The model under review builds one solid part; all positions refer to its coordinate system, in mm. A direction names the side the tool comes from. Round coordinates to 2 decimals unless told otherwise and drop trailing zeros. Loops run counter-clockwise (first coordinate to the right, second up) from the corner with the lowest first, then second, coordinate; pieces in that order, holes last. Notation, with made-up numbers: (-4, 13) -> (44, 13) arc R7 cw to (44, 25) -> close; hole circle Ø11 at (-24.75, 45). An arc over 180 degrees is marked (long way). Use a Markdown table: item, result. Add a question column.
1) Wall thickness on probe 1 along X at (y, z) = (-26, 2.25); probe 2 along X at (y, z) = (-8.5, 12.75); probe 3 along Z at (x, y) = (15, -3.05): over which ranges is each line inside the solid? List them lowest first.
2) Consider section C-C on x = 15. Give the boundary of the cut face in (y, z).
3) Mouldability with a two-part tool opening along X and no side actions: class faces 1 (the flat face through (124, -51, 10)), 2 (the cylindrical face through (2, -5, 10)), 3 (the flat face through (156.735, -22.185, 17.215)), 4 (the flat face through (90, -23, 10)) as released by +X, released by -X, zero draft, split by the parting line, or undercut.
4) Insertion check: pin 1 (8 mm diameter, centred on x = 60, z = 10.26, fed in from -Y); pin 2 (12 mm diameter, centred on y = -8.5, z = 3, fed in from -X); pin 3 (5 mm diameter, centred on y = -12.5, z = 3.5, fed in from -X). Each pin has a flat end and moves straight along its axis. Give the tip position at first contact, or say it passes through.
5) For faces 5 (the flat face through (92.535, -22.815, 17.285)), 6 (the flat face through (95, -23, 3)), 7 (the flat face through (44, -6, 5)), list the 3-axis set-ups (+Z, -Z, +X, -X, +Y, -Y) from which the entire face can be reached by the end or side of a thin tool; tool diameter is ignored.
6) Consider section B-B on z = 1.5. Give the boundary of the cut face in (x, y), plus the area to 3 significant figures.
7) Consider section D-D on x = 81.5. Give the boundary of the cut face in (y, z).
from build123d import *

# Parameters (mm, degrees)
F1_DEPTH    = 20
F3_D        = 6.2484
F4_W        = 45
F4_H        = 6.15
F4_H_2      = 5.25
F6_DEPTH    = 5
F5_W        = 45
F5_H        = 6.15
F5_H_2      = 5.25
F7_DEPTH    = 5
F8_SIZE     = 4.99999
F9_T1_DEPTH = 45
F10_R       = 5


# Not quite as in the source:
# - a fillet or chamfer that OpenCascade refuses, or shapes differently, is made with other operations: its cross-section is extruded or revolved along the edge and cut away or added
# - a fillet or chamfer is up to 0.001 mm smaller than in the source, because OpenCascade refuses the exact size


with BuildPart() as f1:
    # F0 (on Top) → F1 (new body)
    with BuildSketch(Plane.XY):
        Polygon((90, 0), (0, 0), (0, -6), (84, -6), (84, -51), (90, -51), (165.2, -51), (165.2, -45), (165.2, 0), (159.2, 0), (159.2, -45), (90, -45), align=None)
    extrude(amount=F1_DEPTH)

    # F3 (through all)
    with Locations(Plane(origin=(0, 0, 0), x_dir=(-1, 0, 0), z_dir=(0, 1, 0))):
        with Locations((-45, 10.2648036554), (-30, 10.2648036554), (-15, 10.2648036554), (-60, 10.2648036554)):
            Hole(F3_D / 2)

    # F4 (on face) → F6 (join)
    with BuildSketch(Plane(origin=(159.2, 0, 0), x_dir=(0, -1, 0), z_dir=(-1, 0, 0))):
        with Locations((22.5, 3.075)):
            Rectangle(F4_W, F4_H)
        with Locations((22.5, 17.375)):
            Rectangle(F4_W, F4_H_2)
    extrude(amount=F6_DEPTH)

    # F5 (on face) → F7 (join)
    with BuildSketch(Plane.YZ.offset(90)):
        with Locations((-22.5, 3.075)):
            Rectangle(F5_W, F5_H)
        with Locations((-22.5, 17.375)):
            Rectangle(F5_W, F5_H_2)
    extrude(amount=F7_DEPTH)

    # F8 (size 5 in the source; OpenCascade refuses exactly that, so slightly less here)
    f8_edges = [f1.edges().sort_by_distance(p)[0] for p in [
        (154.2, -22.5, 14.75),
        (95, -22.5, 14.75),
    ]]
    chamfer(f8_edges, length=F8_SIZE)

    # F9: fillet of radius 5 on 4 edges, made by hand

    # F9_s2 → F9_t1 (cut)
    with BuildSketch(Plane.XY.offset(-12.5)):
        with BuildLine():
            ThreePointArc((160.2, -51), (163.7355339059, -49.5355339059), (165.2, -46))
            Line((165.2, -46), (165.2, -51))
            Line((165.2, -51), (160.2, -51))
        make_face()
        with BuildLine():
            ThreePointArc((84, -46), (85.4644660941, -49.5355339059), (89, -51))
            Line((89, -51), (84, -51))
            Line((84, -51), (84, -46))
        make_face()
        with BuildLine():
            ThreePointArc((5, 0), (1.4644660941, -1.4644660941), (0, -5))
            Line((0, -5), (0, 0))
            Line((0, 0), (5, 0))
        make_face()
        with BuildLine():
            ThreePointArc((0, -1), (1.4644660941, -4.5355339059), (5, -6))
            Line((5, -6), (0, -6))
            Line((0, -6), (0, -1))
        make_face()
    extrude(amount=F9_T1_DEPTH, mode=Mode.SUBTRACT)

    # F10
    f10_edges = [f1.edges().sort_by_distance(p)[0] for p in [
        (165.2, 0, 10),
    ]]
    fillet(f10_edges, radius=F10_R)


solid = f1.part
Result set:
| question | item | result |
|---|---|---|
| 1 | probe 1 | 84 to 95, 154.2 to 165.2 |
| 1 | probe 2 | 84 to 90, 159.2 to 165.2 |
| 1 | probe 3 | 0 to 7.14, 13.39 to 20 |
| 2 | outline | (-6, 0) -> (0, 0) -> (0, 7.14) -> (-6, 7.14) -> close; (-6, 13.39) -> (0, 13.39) -> (0, 20) -> (-6, 20) -> close |
| 3 | face 1 | zero draft |
| 3 | face 2 | released by -X |
| 3 | face 3 | undercut |
| 3 | face 4 | undercut |
| 4 | pin 1 | y = -6 |
| 4 | pin 2 | x = 0.42 |
| 4 | pin 3 | x = 84 |
| 5 | face 5 | +Y |
| 5 | face 6 | +Z, -Z, +Y |
| 5 | face 7 | +Z, -Z, -X, -Y |
| 6 | outline | (0.42, -3) arc R5 ccw to (5, -6) -> (84, -6) -> (84, -46) arc R5 ccw to (89, -51) -> (160.2, -51) arc R5 ccw to (165.2, -46) -> (165.2, -5) arc R5 ccw to (160.2, 0) -> (154.2, 0) -> (154.2, -45) -> (95, -45) -> (95, 0) -> (5, 0) arc R5 ccw to start |
| 6 | area | 1,950 mm2 |
| 7 | outline | (-6, 0) -> (0, 0) -> (0, 20) -> (-6, 20) -> close |
